Part print with two shaded views. Sizes in mm from the minimum x, y, z corner. Round coordinates to 2 decimals unless told otherwise and drop trailing zeros. Order: outer loops, then holes, each group sorted by start corner. A loop starts at its lowest first (then second) coordinate and runs counter-clockwise, first axis right, second up. Notation, with made-up numbers: (18.5, 29) - (45.5, 29) arc R22 ccw to (45.5, 45) - close; hole circle Ø11 at (-35.75, 74.5). An arc over 180 degrees is marked (long way). Use one line per item in the form item = value.
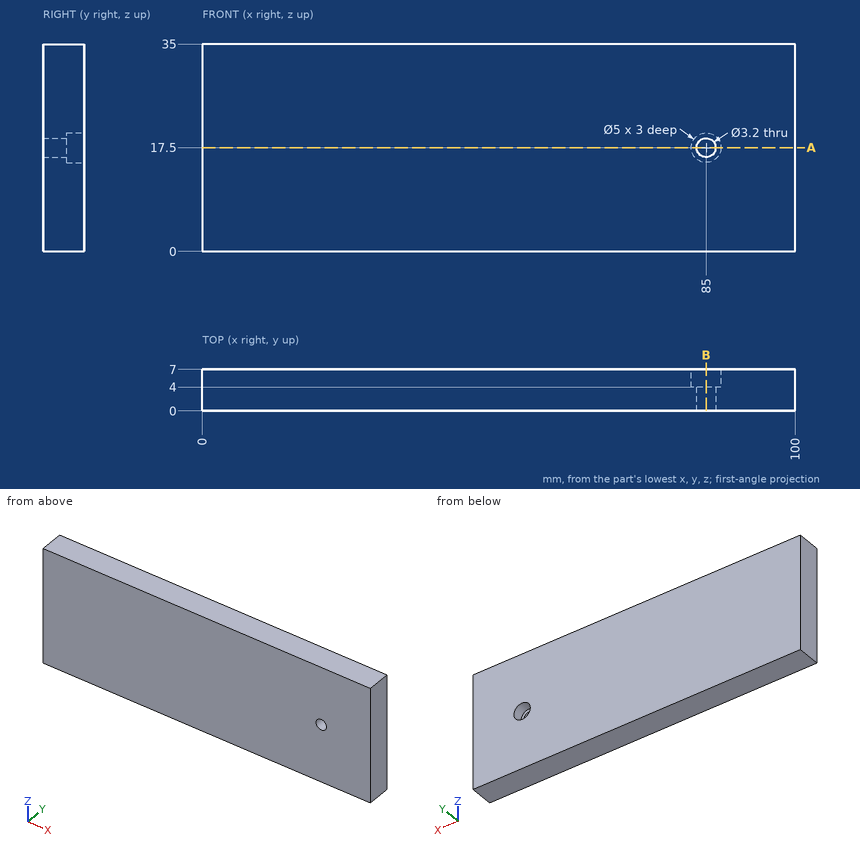
(1) Pin check, flat tip, straight feed: pin 1 (2.5 mm diameter, centred on x = 85, z = 18.5, fed in from +Y). Stop position of the tip, or through.
Report:
pin_1 = 4
(2) Probe probe 1 along Z at (x, y) = (85, 1); probe 2 along X at (y, z) = (1, 17.5); probe 3 along X at (y, z) = (5.45, 17.5). List the from-to ranges inside material, lowest first. Write a range as [from, to].
Report:
probe_1 = [0, 15.9], [19.1, 35]
probe_2 = [0, 83.4], [86.6, 100]
probe_3 = [0, 82.5], [87.5, 100]
(3) Slice it at A-A on z = 17.5. Give the cut face in (x, y), then the cut area to 3 significant figures.
Report:
outline = (0, 0) - (83.4, 0) - (83.4, 4) - (82.5, 4) - (82.5, 7) - (0, 7) - close; (86.6, 0) - (100, 0) - (100, 7) - (87.5, 7) - (87.5, 4) - (86.6, 4) - close
area = 672 mm2
(4) Slice it at B-B on x = 85. Give the cut face in (y, z), then the cut area to 3 significant figures.
Report:
outline = (0, 0) - (7, 0) - (7, 15) - (4, 15) - (4, 15.9) - (0, 15.9) - close; (0, 19.1) - (4, 19.1) - (4, 20) - (7, 20) - (7, 35) - (0, 35) - close
area = 217 mm2
